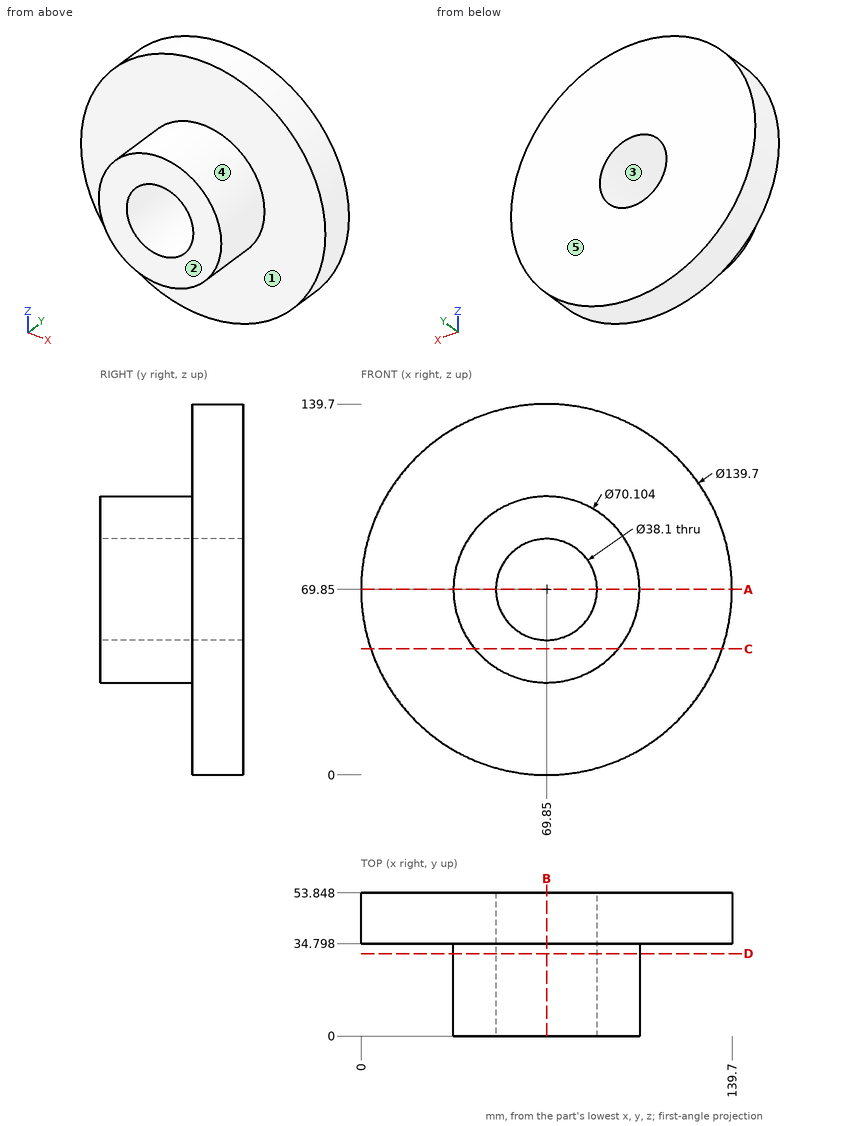
Answer from the drawing. Dimensions are ordinates in mm from the lowest x, y and z of the part. A direction names the side the tool comes from. Coordinates: 2 decimals unless noted, no trailing zeros. Loops run counter-clockwise (first coordinate to the right, second up) from the corner with the lowest first, then second, coordinate; pieces in that order, holes last.
1) Flat-ended cylindrical pins translate along their axes: pin 1 (1 mm diameter, centred on x = 31, y = 34, fed in from -Z); pin 2 (2 mm diameter, centred on x = 88, y = 18.5, fed in from +Z); pin 3 (5 mm diameter, centred on y = 37.5, z = 62.5, fed in from +X); pin 4 (3 mm diameter, centred on y = 29.5, z = 76, fed in from -X). Find the tip coordinate at first contact, or state that the pin passes through.
Results:
pin 1: passes through
pin 2: stops at z = 100.42
pin 3: stops at x = 139.53
pin 4: stops at x = 35.11
2) For a pull along X with two mould halves and no side action, classify the marked faces 3, 4 and 5 as +X half, -X half, draft (parallel to the pull), parting line (faces both ways), or undercut.
Results:
face 3: undercut
face 4: parting line
face 5: draft
3) Consider probe 1 along Z at (x, y) = (69, 34); probe 2 along Z at (x, y) = (69.85, 36). Determine where each line is inside the solid, lowest interval first.
Results:
probe 1: z = 34.81 to 50.82, 88.88 to 104.89
probe 2: z = 0 to 50.8, 88.9 to 139.7
4) Section B-B (x = 69.85) is taken. Give the vertices of the cut face in (y, z), plus the area to 3 significant figures.
Results:
outline: (0, 34.8) - (34.8, 34.8) - (34.8, 0) - (53.85, 0) - (53.85, 50.8) - (0, 50.8) - close; (0, 88.9) - (53.85, 88.9) - (53.85, 139.7) - (34.8, 139.7) - (34.8, 104.9) - (0, 104.9) - close
area: 3,050 mm2
5) Section D-D (y = 31) is taken. Give the vertices of the cut face in (x, z), plus the area to 3 significant figures.
Results:
outline: circle Ø70.1 at (69.85, 69.85); hole circle Ø38.1 at (69.85, 69.85)
area: 2,720 mm2
6) Section A-A (z = 69.85) is taken. Give the vertices of the cut face in (x, y), plus the area to 3 significant figures.
Results:
outline: (0, 34.8) - (34.8, 34.8) - (34.8, 0) - (50.8, 0) - (50.8, 53.85) - (0, 53.85) - close; (88.9, 0) - (104.9, 0) - (104.9, 34.8) - (139.7, 34.8) - (139.7, 53.85) - (88.9, 53.85) - close
area: 3,050 mm2
7) For the marked faces 1 and 2, determine the directions among +Z, -Z, +X, -X, +Y, -Y from which every point of the face is accessible in a straight line to the end or side of a thin tool.
Results:
face 1: -Y
face 2: +Z, -Z, +X, -X, -Y
8) Section C-C (z = 47.5) is taken. Give the vertices of the cut face in (x, y), plus the area to 3 significant figures.
Results:
outline: (3.67, 34.8) - (42.85, 34.8) - (42.85, 0) - (96.85, 0) - (96.85, 34.8) - (136.03, 34.8) - (136.03, 53.85) - (3.67, 53.85) - close
area: 4,400 mm2
